The model under review builds one solid part; all positions refer to its coordinate system, in mm. Round coordinates to 2 decimals unless told otherwise and drop trailing zeros. Write each loop counter-clockwise with the first axis right and the second up, starting at its lowest first coordinate (ties: lowest second). Pieces come first, ordered by that corner, then holes. Notation, with made-up numbers: M 61.5,26 L 65.5,26 A23 ccw 65.5,54 Z; hole C -17.5,44.25 d1. An arc over 180 degrees is marked long. Write item = value, one per line. Start each with the question number.
Item 1: Take a section at C-C, the plane x = 44.5. Give the boundary of the cut face in (y, z), plus the area to 3 significant figures.
Item 2: To check wall thickness, follow line 1 along Z through (x, y) = (-29.5, 0.55); line 2 along X through (y, z) = (1.2, 35); line 3 along X through (y, z) = (0.95, 34). State the ranges of each line that lie inside material, in increasing order.
Item 3: Take a section at B-B, the plane z = 45.5. Give the boundary of the cut face in (x, y), plus the area to 3 significant figures.
Item 4: Take a section at A-A, the plane y = 0.6. Give the boundary of the cut face in (x, z), plus the area to 3 significant figures.
Item 5: For pin 1 Ø1.8 at (x, z) = (28.95, -34.5) entering from +Y, flat-tipped, find the tip position at first contact; note if it passes through.
Item 6: The part is to be moulded in two halves that separate along X. For faces 1 (the cylindrical face through (29.404, 0.811, -33.074)), 2 (the flat face through (61.127, 0.789, -10.623)), 3 (the flat face through (-21.076, 0.789, -58.354)), say which applies: +X half, -X half, draft (parallel to the pull), parting line (faces both ways), or undercut.
from build123d import *

# Parameters (mm, degrees)
BOSS_EXTRUDE1_DEPTH = 1.6
SKETCH7_R           = 1.5
CUT_EXTRUDE4_DEPTH  = 1.6


with BuildPart() as part:
    # Sketch1 → Boss-Extrude1 (new body)
    with BuildSketch(Plane(origin=(0, 0, 0), x_dir=(1, 0, 0), z_dir=(0, 1, 0))):
        Polygon((63, 0), (59.20063511, 21.54726903), (48.260799916, 40.49561941), (31.5, 54.559600438), (10.939835193, 62.04288844), (-10.939835193, 62.04288844), (-31.5, 54.559600438), (-48.260799916, 40.49561941), (-59.20063511, 21.54726903), (-63, 0), (-59.20063511, -21.54726903), (-48.260799916, -40.49561941), (-31.5, -54.559600438), (-10.939835193, -62.04288844), (10.939835193, -62.04288844), (31.5, -54.559600438), (48.260799916, -40.49561941), (59.20063511, -21.54726903), align=None)
    extrude(amount=BOSS_EXTRUDE1_DEPTH)

    # Sketch7 → Cut-Extrude4 (cut)
    with BuildSketch(Plane(origin=(0, 1.6, 0), x_dir=(1, 0, 0), z_dir=(0, 1, 0))):
        with Locations(Location((-28.953010594, 34.504854391, 0), (0, 0, 270))):
            Circle(SKETCH7_R)
        with Locations(Location((28.953010594, 34.504854391, 0), (0, 0, 270))):
            Circle(SKETCH7_R)
        with Locations(Location((-28.953010594, -34.504854391, 0), (0, 0, 270))):
            Circle(SKETCH7_R)
        with Locations(Location((28.953010594, -34.504854391, 0), (0, 0, 270))):
            Circle(SKETCH7_R)
    extrude(amount=-CUT_EXTRUDE4_DEPTH, mode=Mode.SUBTRACT)


solid = part.part
Response values:
q1.outline = M 0,-43.65 L 1.6,-43.65 L 1.6,43.65 L 0,43.65 Z
q1.area = 140 mm2
q2.line_1 = -55.29 to -35.9, -33.11 to 33.11, 35.9 to 55.29
q2.line_2 = -51.43 to -30.37, -27.54 to 27.54, 30.37 to 51.43
q2.line_3 = -52.01 to -30.37, -27.54 to 27.54, 30.37 to 52.01
q3.outline = M -42.3,0 L 42.3,0 L 42.3,1.6 L -42.3,1.6 Z
q3.area = 135 mm2
q4.outline = M -63,0 L -59.2,-21.55 L -48.26,-40.5 L -31.5,-54.56 L -10.94,-62.04 L 10.94,-62.04 L 31.5,-54.56 L 48.26,-40.5 L 59.2,-21.55 L 63,0 L 59.2,21.55 L 48.26,40.5 L 31.5,54.56 L 10.94,62.04 L -10.94,62.04 L -31.5,54.56 L -48.26,40.5 L -59.2,21.55 Z; hole C -28.95,-34.5 d3; hole C -28.95,34.5 d3; hole C 28.95,-34.5 d3; hole C 28.95,34.5 d3
q4.area = 12,200 mm2
q5.pin_1 = through
q6.face_1 = undercut
q6.face_2 = +X half
q6.face_3 = -X half
